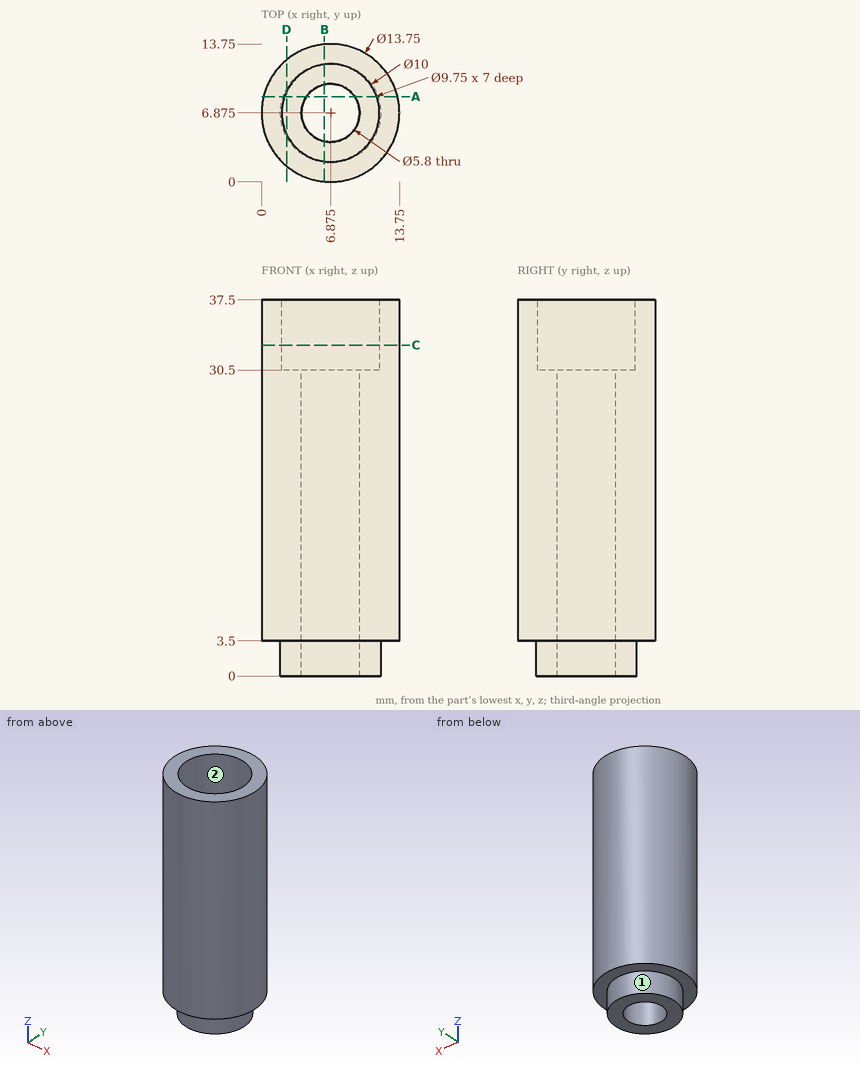
Study the drawing (mm; zero at the part's minimum x, y, z) and answer. Coordinates: 2 decimals unless noted, no trailing zeros. Loops run counter-clockwise (first coordinate to the right, second up) from the corner with the lowest first, then second, coordinate; pieces in that order, holes last. Notation, with made-up numbers: (23, -7) -> (77, -7) arc R26 cw to (77, 14) -> close; hole circle Ø1 at (-21.75, -3). An arc over 180 degrees is marked (long way). Write each question's results on one line, items separated by ' | '. Start each with the question number.
1) Find section B-B on x = 6.25. Determine the outline of the cut face in (y, z), then the cut area to 3 significant figures.
2) Flat-ended cylindrical pins translate along their axes: P1, Ø4, axis at x = 3, z = 5.5, coming from the +Y side; P2, Ø3, axis at y = 11, z = 13, coming from the +X side; P3, Ø1.5, axis at x = 1.5, z = 27.5, coming from the +Y side; P4, Ø8, axis at x = 6, y = 8, coming from the +Z side. Find the tip coordinate at first contact, or state that the pin passes through.
3) The mould has two halves that part along X. Classify the marked faces 1 and 2: pulls with the +X half, pulls with the -X half, needs draft (parallel to the pull), parting line crosses it, or undercut.
4) Find section C-C on z = 33. Determine the outline of the cut face in (x, y) (3 decimals).
5) Find section D-D on x = 2.5. Determine the outline of the cut face in (y, z).
6) Find section A-A on y = 8.5. Determine the outline of the cut face in (x, z), then the cut area to 3 significant figures.
7) Consider line 1 along X through (y, z) = (7, 23); line 2 along Z through (x, y) = (4, 4.75); line 3 along X through (y, z) = (6.75, 2.5). Determine where each line is inside the solid, lowest interval first.
Response values:
1) outline: (0.03, 3.5) -> (1.91, 3.5) -> (1.91, 0) -> (4.04, 0) -> (4.04, 30.5) -> (2.04, 30.5) -> (2.04, 37.5) -> (0.03, 37.5) -> close; (9.71, 0) -> (11.84, 0) -> (11.84, 3.5) -> (13.72, 3.5) -> (13.72, 37.5) -> (11.71, 37.5) -> (11.71, 30.5) -> (9.71, 30.5) -> close | area: 260 mm^2
2) P1: stops at y = 13.49 | P2: stops at x = 13.23 | P3: stops at y = 11.96 | P4: stops at z = 37.5
3) face 1: parting line crosses it | face 2: undercut
4) outline: circle Ø13.75 at (6.875, 6.875); hole circle Ø9.75 at (6.875, 6.875)
5) outline: (1.57, 3.5) -> (4.45, 3.5) -> (4.45, 0) -> (9.3, 0) -> (9.3, 3.5) -> (12.18, 3.5) -> (12.18, 37.5) -> (9.03, 37.5) -> (9.03, 30.5) -> (4.72, 30.5) -> (4.72, 37.5) -> (1.57, 37.5) -> close
6) outline: (0.19, 3.5) -> (2.15, 3.5) -> (2.15, 0) -> (4.47, 0) -> (4.47, 30.5) -> (2.28, 30.5) -> (2.28, 37.5) -> (0.19, 37.5) -> close; (9.28, 0) -> (11.6, 0) -> (11.6, 3.5) -> (13.56, 3.5) -> (13.56, 37.5) -> (11.47, 37.5) -> (11.47, 30.5) -> (9.28, 30.5) -> close | area: 276 mm^2
7) line 1: x = 0 to 3.98, 9.77 to 13.75 | line 2: z = 0 to 30.5 | line 3: x = 1.88 to 3.98, 9.77 to 11.87
